Autodesk Inventor part; units mm, degrees
ref_plane "工作平面1" through (750, 0, 0) normal (1, 0, 0) x (0, 0, -1)
ref_plane "YZ Plane" through (0, 0, 0) normal (1, 0, 0) x (0, 1, 0)
ref_plane "XZ Plane" through (0, 0, 0) normal (0, 1, 0) x (-1, 0, 0)
sketch "草圖1" plane through (0, 0, 0) normal (1, 0, 0) x (0, 1, 0)
  line L0 (500, 1000) -> (500, -1000)
  line L1 (0, 650) -> (0, -650)
  line L2 (0, -650) -> (500, -1000)
  line L3 (0, 650) -> (500, 1000)
  line L4 (500, 1000) -> (700, 1000)
  line L5 (700, 1000) -> (700, -1000)
  line L6 (700, -1000) -> (500, -1000)
  line L7 (500, -1000) -> (500, 1000)
  circle A0 centre (560, 875) radius 90
  line L8 (785.0874, 735) -> (28.1159, 735)
  point P0 (0, 0)
  point P1 (0, 0)
  point P2 (500, 0)
  point P3 (700, 735)
  point P4 (560, 785)
  point P5 (121.4286, 735)
  point P6 (500, 735)
  point P7 (500, 807.918)
  point P8 (500, 942.082)
  dimension "d0" = 1300
  dimension "d1" = 2000
  dimension "d2" = 500
  dimension "d3" = 200
  dimension "d6" = 180
  dimension "d7" = 140
  dimension "d8" = 125
  dimension "d32" = 265
extrude "擠出1" add sketch "草圖1" along normal mid plane 1700 contours A0 L0 | L0 A0 | L8 L0 L2 L1 L3 | L8 L5 L6 L0
extrude "擠出2" add sketch "草圖1" against normal blind 500 from surface at 850 contours L4 L5 L8 L0 A0 | L0 A0 L8 L3 | A0 L0 | L0 A0 | L8 L0 L2 L1 L3
extrude "擠出3" add sketch "草圖1" along normal blind 500 from surface at -850 contours L4 L5 L8 L0 A0 | L0 A0 L8 L3 | A0 L0 | L0 A0 | L8 L0 L2 L1 L3
sketch "草圖2" plane through (-350, 560, 875) normal (1, 0, 0) x (0, 0, -1)
  circle A0 centre (10, -180) radius 22.5
  line L0 (140, -438.5714) -> (140, 140)
  line L1 (-125, 140) -> (140, 140)
  line L2 (-125, -60) -> (-125, 140)
  line L3 (140, -438.5714) -> (-125, -60)
  line L4 (225, -560) -> (140, -438.5714)
  line L5 (1525, -560) -> (225, -560)
  line L6 (1875, -60) -> (1525, -560)
  line L7 (1875, 140) -> (1875, -60)
  line L8 (140, 140) -> (1875, 140)
  circle A1 centre (0, 0) radius 90
  point P0 (875, -560)
  dimension "d13" = 45
  dimension "d15" = 320
extrude "擠出4" add sketch "草圖2" along normal up to next contours A0
ref_plane "工作平面1" through (750, 0, 0) normal (1, 0, 0) x (0, 0, -1)
sketch "草圖4" plane through (750, 0, 0) normal (1, 0, 0) x (0, 0, -1)
  line L0 (-1000, 700) -> (1000, 700)
  line L1 (1000, 700) -> (1000, 500)
  line L2 (1000, 500) -> (650, 0)
  line L3 (650, 0) -> (-650, 0)
  line L4 (-650, 0) -> (-1000, 500)
  line L5 (-1000, 500) -> (-1000, 700)
  line L6 (597.9344, 100) -> (900, 531.5222)
  line L7 (900, 531.5222) -> (900, 600)
  line L8 (900, 600) -> (-900, 600)
  line L9 (-900, 600) -> (-900, 531.5222)
  line L10 (-900, 531.5222) -> (-597.9344, 100)
  line L11 (-597.9344, 100) -> (597.9344, 100)
  line L12 (-597.9344, 1100.1132) -> (-597.9344, -380.0313)
  point P0 (0, 0)
  point P1 (-597.9344, 600)
  dimension "d20" = 100
extrude "擠出5" cut sketch "草圖4" against normal blind 1500 contours L8 L7 L6 L11 L12
sketch "草圖5" plane through (850, 0, 0) normal (1, 0, 0) x (0, 0, -1)
  circle A0 centre (-547.9344, 150) radius 50
  circle A1 centre (571.9017, 150) radius 50
  line L0 (-650, 0) -> (650, 0)
  line L1 (-597.9344, 600) -> (-597.9344, 100)
  line L2 (-597.9344, 100) -> (597.9344, 100)
  line L3 (597.9344, 100) -> (900, 531.5222)
  point P0 (0, 0)
  dimension "d24" = 100
  dimension "d25" = 100
extrude "擠出6" cut sketch "草圖5" against normal through all contours A0 | A1
thread "螺紋2"
equation "\"d25\" = d24"
properties part number "車身"
Work out the finished part from the listing and answer in its coordinate system (mm). A direction names the side the tool comes from. Coordinates: 2 decimals unless noted, no trailing zeros. Write each loop counter-clockwise with the first axis right and the second up, starting at its lowest first coordinate (ties: lowest second). Pieces come first, ordered by that corner, then holes. Notation, with made-up numbers: M -13,-19.5 L 21,-19.5 A25 ccw 21,9.5 Z; hole C -34,79 d3. An arc over 180 degrees is marked long. Use one line per item in the form item = value. Start each with the question number.
1. Each of these flat-tipped pins is pushed along its axis until it touches: P1, Ø3, axis at x = 594, z = 104, coming from the -Y side; P2, Ø8, axis at x = 95, y = 253.5, coming from the -Z side; P3, Ø2, axis at x = 594, y = 313, coming from the +Z side. Where does it stop, or does it pass through?
2. The mould has two halves that part along X. Classify faces 3 (the face through (850, 345, 14)), 4 (the face through (-750, 112, 588)), 5 (the face through (-604, 599, 1000)): released by +X, released by -X, zero draft, split by the parting line, or undercut.
3. Straight lines are drawn through the part: probe 1 along Y at (x, z) = (-254.5, -125.5); probe 2 along X at (y, z) = (547.5, -41); probe 3 along X at (y, z) = (208, 789). For each, find the intervals that lie inside material, in ascending order. Write a range as from..to.
4. A tool of negligible diameter and unlimited length cuts with its end or side. For faces 1 (the face through (750, 354, -141)), 2 (the face through (-12, 80, 706)), from which of +Z, -Z, +X, -X, +Y, -Y can it reach the whole face along a straight path? Write none if from no direction.
5. The part is cut by section D-D (y = 266). Give the vertices of the cut face in (x, z), plus the area to 3 significant figures.
6. The part is cut by section B-B (x = -624). Give the vertices of the cut face in (y, z).
7. The part is cut by section C-C (z = -121). Give the vertices of the cut face in (x, y), plus the area to 3 significant figures.
8. The part is cut by section A-A (y = 560). Give the vertices of the cut face in (x, z).
Evaluation:
q1.P1 = 0
q1.P2 = -830.25
q1.P3 = 869.8
q2.face_3 = released by +X
q2.face_4 = undercut
q2.face_5 = zero draft
q3.probe_1 = 0..100, 600..700
q3.probe_2 = -850..-750, 750..850
q3.probe_3 = -850..-350, 350..850
q4.face_1 = none
q4.face_2 = +Z, +X, -X, -Y
q5.outline = M -850,-836.2 L 850,-836.2 L 850,836.2 L 350,836.2 L 350,735 L -350,735 L -350,836.2 L -850,836.2 Z; hole M -750,-714.13 L 750,-714.13 L 750,597.93 L -750,597.93 Z
q5.area = 804,000 mm^2
q6.outline = M 0,-650 L 500,-1000 L 700,-1000 L 700,1000 L 500,1000 L 0,650 Z; hole M 100,-597.93 L 121.26,-612.82 A50 ccw 121.39,-612.91 L 531.52,-900 L 600,-900 L 600,597.93 L 100,597.93 Z
q7.outline = M -850,0 L 850,0 L 850,700 L -850,700 Z; hole M -750,100 L 750,100 L 750,600 L -750,600 Z
q7.area = 440,000 mm^2
q8.outline = M -850,-1000 L 850,-1000 L 850,1000 L 350,1000 L 350,965 L -350,965 L -350,1000 L -850,1000 Z; hole M -750,-900 L 750,-900 L 750,597.93 L -750,597.93 Z; hole M -350,735 L 350,735 L 350,785 L -350,785 Z
